Build history of the part. All positions in model axes, mm. Coordinates: 2 decimals unless noted, no trailing zeros. Loops run counter-clockwise (first coordinate to the right, second up) from the corner with the lowest first, then second, coordinate; pieces in that order, holes last. Notation, with made-up numbers: M 72,-18 L 116,-18 A10 cw 116,-7 Z; hole C 51.5,32.5 d10. An arc over 180 degrees is marked long. Write each question's results on one line, items separated by ' | '. Start each with the question number.
from build123d import *

# Parameters (mm, degrees)
SKETCH1_R               = 43.5
SKETCH1_R_2             = 33.5
BOSS_EXTRUDE1_DEPTH     = 3
SKETCH3_R               = 2.025
CUT_EXTRUDE2_DEPTH      = 62.591395503
CIRPATTERN1_COUNT       = 12
CUT_EXTRUDE1_DEPTH      = 62.591395503
BOSS_EXTRUDE2_DEPTH     = 3
CUT_EXTRUDE_THIN1_DEPTH = 3
FILLET1_R               = 1.2
FILLET2_R               = 5
CUT_EXTRUDE3_DEPTH      = 112.227677485
CUT_EXTRUDE3_DEPTH_BACK = 112.227677485
SKETCH6_R               = 2.525


with BuildPart() as part:
    # Sketch1 → Boss-Extrude1 (new body)
    with BuildSketch(Plane(origin=(0, 0, 0), x_dir=(1, 0, 0), z_dir=(0, 1, 0))):
        with Locations(Location((0, 0, 0), (0, 0, 270))):
            Circle(SKETCH1_R)
        with Locations(Location((0, 0, 0), (0, 0, 270))):
            Circle(SKETCH1_R_2, mode=Mode.SUBTRACT)
    extrude(amount=BOSS_EXTRUDE1_DEPTH)

    # Sketch3 → Cut-Extrude2 (cut, symmetric)
    with BuildSketch(Plane(origin=(0, 3, 0), x_dir=(1, 0, 0), z_dir=(0, 1, 0))):
        with Locations(Location((-38, 0, 0), (0, 0, 270))):
            Circle(SKETCH3_R)
    cut_extrude2 = extrude(amount=CUT_EXTRUDE2_DEPTH, both=True, mode=Mode.SUBTRACT)

    # CirPattern1: Cut-Extrude2 ×12 about axis
    cirpattern1_axis = Axis((0, 0, 0), (0, 1, 0))
    for i in range(1, CIRPATTERN1_COUNT):
        add(cut_extrude2.rotate(cirpattern1_axis, i * 360 / CIRPATTERN1_COUNT), mode=Mode.SUBTRACT)

    # Sketch2 → Cut-Extrude1 (cut, symmetric)
    with BuildSketch(Plane(origin=(0, 3, 0), x_dir=(1, 0, 0), z_dir=(0, 1, 0))):
        with BuildLine():
            Line((0, 0), (43.5, 0))
            ThreePointArc((43.5, 0), (24.950574981, -35.633113927), (-14.877876235, -40.876629004))
            Line((-14.877876235, -40.876629004), (0, 0))
        make_face()
    cut_extrude1 = extrude(amount=CUT_EXTRUDE1_DEPTH, both=True, mode=Mode.SUBTRACT)

    # Mirror1: Cut-Extrude1 across plane
    add(cut_extrude1.mirror(Plane.XY), mode=Mode.SUBTRACT)

    # Sketch4 → Boss-Extrude2 (add)
    with BuildSketch(Plane(origin=(0, 0, 0), x_dir=(1, 0, 0), z_dir=(0, 1, 0))):
        with BuildLine():
            ThreePointArc((-30.759144982, -30.759144982), (-35.633113927, -24.950574981), (-39.424388736, -18.383894386))
            Line((-39.424388736, -18.383894386), (-57.550544477, -26.836259621))
            Line((-57.550544477, -26.836259621), (-76.583008005, -35.711243117))
            ThreePointArc((-76.583008005, -35.711243117), (-51.440340751, -67.038357255), (-14.673271013, -83.21625513))
            Line((-14.673271013, -83.21625513), (-11.026659282, -62.535292316))
            ThreePointArc((-11.026659282, -62.535292316), (-29.32103694, -56.325187907), (-44.901280605, -44.901280605))
            Line((-44.901280605, -44.901280605), (-30.759144982, -30.759144982))
        make_face()
    extrude(amount=BOSS_EXTRUDE2_DEPTH)

    # Sketch5 → Cut-Extrude-Thin1 (cut)
    with BuildSketch(Plane(origin=(0, 3, 0), x_dir=(1, 0, 0), z_dir=(0, 1, 0))):
        with BuildLine():
            ThreePointArc((-46.972968566, -52.168766749), (-32.414752649, -62.268160489), (-15.791564015, -68.400778548))
            Line((-15.791564015, -68.400778548), (-15.251681485, -66.062290392))
            ThreePointArc((-15.251681485, -66.062290392), (-31.306555977, -60.139334489), (-45.367055111, -50.385219167))
            Line((-45.367055111, -50.385219167), (-46.972968566, -52.168766749))
        make_face()
        with BuildLine():
            ThreePointArc((-53.329709327, -59.228642591), (-36.801364475, -70.694763404), (-17.928599031, -77.657294163))
            Line((-17.928599031, -77.657294163), (-17.388716501, -75.318806008))
            ThreePointArc((-17.388716501, -75.318806008), (-35.693167803, -68.565937405), (-51.723795872, -57.445095009))
            Line((-51.723795872, -57.445095009), (-53.329709327, -59.228642591))
        make_face()
    extrude(amount=-CUT_EXTRUDE_THIN1_DEPTH, mode=Mode.SUBTRACT)

    # Fillet1
    fillet1_edges = [part.edges().sort_by_distance(p)[0] for p in [
        (-46.972968566, 1.5, 52.168766749),
        (-53.329709327, 1.5, 59.228642591),
        (-45.367055111, 1.5, 50.385219167),
        (-51.723795872, 1.5, 57.445095009),
        (-15.251681485, 1.5, 66.062290392),
        (-17.388716501, 1.5, 75.318806008),
        (-15.791564015, 1.5, 68.400778548),
        (-17.928599031, 1.5, 77.657294163),
    ]]
    fillet(fillet1_edges, radius=FILLET1_R - 0.0001)  # a hair under: the kernel refuses the full size

    # Fillet2
    fillet2_edges = [part.edges().sort_by_distance(p)[0] for p in [
        (-14.877876235, 1.5, -40.876629004),
        (-11.457674801, 1.5, -31.479702796),
        (-11.457674801, 1.5, 31.479702796),
        (-14.877876235, 1.5, 40.876629004),
        (-39.424388736, 1.5, 18.383894386),
        (-76.583008005, 1.5, 35.711243117),
        (-14.673271013, 1.5, 83.21625513),
        (-11.026659282, 1.5, 62.535292316),
        (-30.759144982, 1.5, 30.759144982),
        (-44.901280605, 1.5, 44.901280605),
    ]]
    fillet(fillet2_edges, radius=FILLET2_R - 0.0001)  # a hair under: the kernel refuses the full size

    # Sketch6 → Cut-Extrude3 (cut, two sides: drawn at the far end of the back side and taken through both)
    with BuildSketch(Plane(origin=(0, 3, 0), x_dir=(1, 0, 0), z_dir=(0, 1, 0)).offset(-CUT_EXTRUDE3_DEPTH_BACK)):
        with Locations(Location((-58.287376448, -35.022589094, 0), (0, 0, 270))):
            Circle(SKETCH6_R)
        with Locations(Location((-66.859049455, -40.172969843, 0), (0, 0, 270))):
            Circle(SKETCH6_R)
    extrude(amount=CUT_EXTRUDE3_DEPTH + CUT_EXTRUDE3_DEPTH_BACK, mode=Mode.SUBTRACT)


solid = part.part
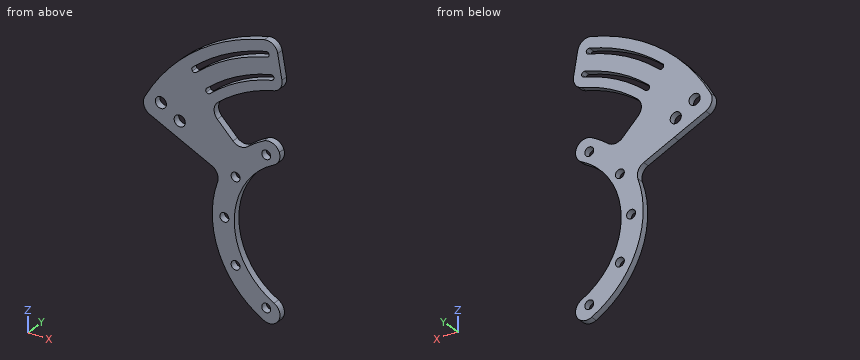
1. Band-saw the part on C-C, the plane z = 63. List the corners of the cut face in (x, y), plus the area to 3 significant figures.
2. Band-saw the part on A-A, the plane z = -19. List the corners of the cut face in (x, y), plus the area to 3 significant figures.
3. Band-saw the part on B-B, the plane x = -38. List the corners of the cut face in (y, z) (1 decimal), plus the area to 3 significant figures.
4. Pin check, flat tips, straight feed: pin 1 (1.5 mm diameter, centred on y = 2, z = -13, fed in from +X); pin 2 (1.5 mm diameter, centred on x = -44, y = 1, fed in from +Z). Stop position of each tip, or through.
5. Wall check: line 1 along Z through (x, y) = (-35.5, 2.65); line 2 along Z through (x, y) = (-16.5, 2.35); line 3 along Z through (x, y) = (-39, 1.6). Give the ranges that are in metal, low to high.
6. Band-saw the part on D-D, the plane y = 1.9. Give the number of separate pieces and of enclosed holes in the cut face, plus the area to 3 significant figures.
Checked values:
1) outline: M -56.31,0 L -48.82,0 L -48.82,3 L -56.31,3 Z; M -44.79,0 L -30.97,0 L -30.97,3 L -44.79,3 Z; M -25.06,0 L -13.13,0 L -13.13,3 L -25.06,3 Z | area: 99.7 mm²
2) outline: M -39.13,0 L -34.93,0 L -34.93,3 L -39.13,3 Z; M -30.88,0 L -27.59,0 L -27.59,3 L -30.88,3 Z | area: 22.5 mm²
3) outline: M 0,-21.2 L 3,-21.2 L 3,-2 L 0,-2 Z; M 0,2 L 3,2 L 3,38 L 0,38 Z; M 0,50.9 L 3,50.9 L 3,56.2 L 0,56.2 Z; M 0,59 L 3,59 L 3,67.3 L 0,67.3 Z; M 0,70.1 L 3,70.1 L 3,75.5 L 0,75.5 Z | area: 222 mm²
4) pin 1: x = -30.55 | pin 2: z = 72.59
5) line 1: -25.14 to 35.5, 52.65 to 57.76, 60.56 to 68.67, 71.36 to 76.68 | line 2: -39 to -29.15, 29.15 to 39, 61.32 to 65.76, 68.14 to 81.76 | line 3: -19.27 to -1.76, 1.76 to 39, 50.11 to 55.46, 58.37 to 66.74, 69.51 to 74.96
6) separate pieces: 1 | enclosed holes: 9 | area: 2,500 mm²
